Answer from the drawing. Dimensions are ordinates in mm from the lowest x, y and z of the part. A direction names the side the tool comes from. Coordinates: 2 decimals unless noted, no trailing zeros. Write each loop counter-clockwise with the first axis right and the second up, starting at its lowest first coordinate (ties: lowest second). Pieces come first, ordered by that corner, then holes.
(1) Which of the six approach directions +Z, -Z, +X, -X, +Y, -Y give full straight-line access (tool end or side, diameter ignored) to the marked faces 4, 5 and 6?
(2) The part is cut by section A-A on y = 34. Determine the outline of the cut face in (x, z), plus the area to 3 significant figures.
(3) Straight lines are drawn through the part: line 1 (Y direction, x = 45, z = 24.5); line 2 (Z direction, x = 80.5, y = 13); line 3 (Z direction, x = 7, y = 35). For each, find the intervals that lie inside material, in ascending order.
(4) The part is cut by section C-C on z = 16. Determine the outline of the cut face in (x, y), plus the area to 3 significant figures.
(5) Given P1, Ø14.5, axis at y = 33, z = 16, coming from the -X side; P2, Ø6.5, axis at x = 8, z = 15, coming from the +Y side; P3, Ø5, axis at y = 56, z = 19, coming from the -X side, each flat-ended and moving along its own axis, determine where each tip first touches the part or whether it passes through.
(6) For a pull along X with two mould halves and no side action, classify the marked faces 1, 2 and 3 as +X half, -X half, draft (parallel to the pull), parting line (faces both ways), or undercut.
(7) The part is cut by section D-D on y = 49.5. Determine the outline of the cut face in (x, z), plus the area to 3 significant figures.
(8) The part is cut by section B-B on x = 80.5. Determine the outline of the cut face in (y, z), plus the area to 3 significant figures.
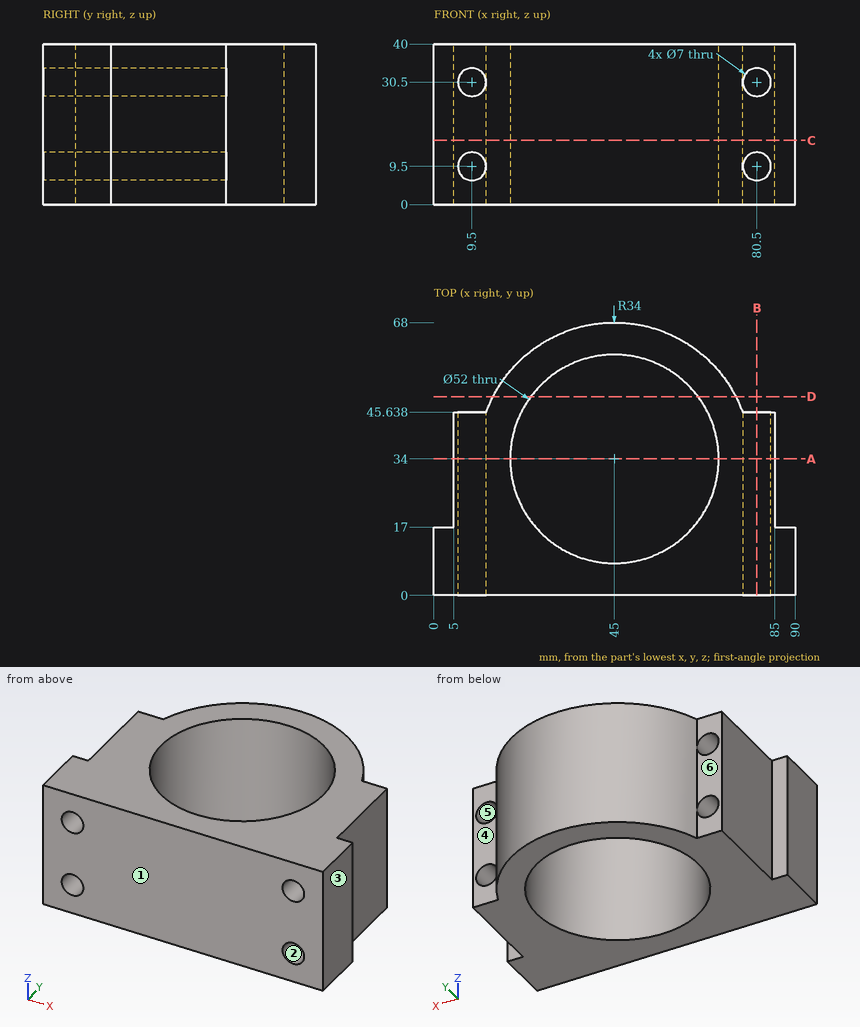
Model answer:
1. face 4: +Z, -Z, +X, +Y
1. face 5: +Y, -Y
1. face 6: +Z, -Z, -X, +Y
2. outline: (5, 0) - (19, 0) - (19, 40) - (5, 40) - close; (71, 0) - (85, 0) - (85, 40) - (71, 40) - close; hole circle Ø7 at (9.5, 9.5); hole circle Ø7 at (9.5, 30.5); hole circle Ø7 at (80.5, 9.5); hole circle Ø7 at (80.5, 30.5)
2. area: 966 mm2
3. line 1: y = 0 to 8, 60 to 68
3. line 2: z = 0 to 6, 13 to 27, 34 to 40
3. line 3: z = 0 to 7.05, 11.95 to 28.05, 32.95 to 40
4. outline: (0, 0) - (90, 0) - (90, 17) - (85, 17) - (85, 45.64) - (76.95, 45.64) arc R34 ccw to (13.05, 45.64) - (5, 45.64) - (5, 17) - (0, 17) - close; hole circle Ø52 at (45, 34)
4. area: 2,740 mm2
5. P1: stops at x = 5
5. P2: stops at y = 45.64
5. P3: stops at x = 17.15
6. face 1: draft
6. face 2: undercut
6. face 3: +X half
7. outline: (14.74, 0) - (24.13, 0) - (24.13, 40) - (14.74, 40) - close; (65.87, 0) - (75.26, 0) - (75.26, 40) - (65.87, 40) - close
7. area: 751 mm2
8. outline: (0, 0) - (45.64, 0) - (45.64, 6) - (0, 6) - close; (0, 13) - (45.64, 13) - (45.64, 27) - (0, 27) - close; (0, 34) - (45.64, 34) - (45.64, 40) - (0, 40) - close
8. area: 1,190 mm2
